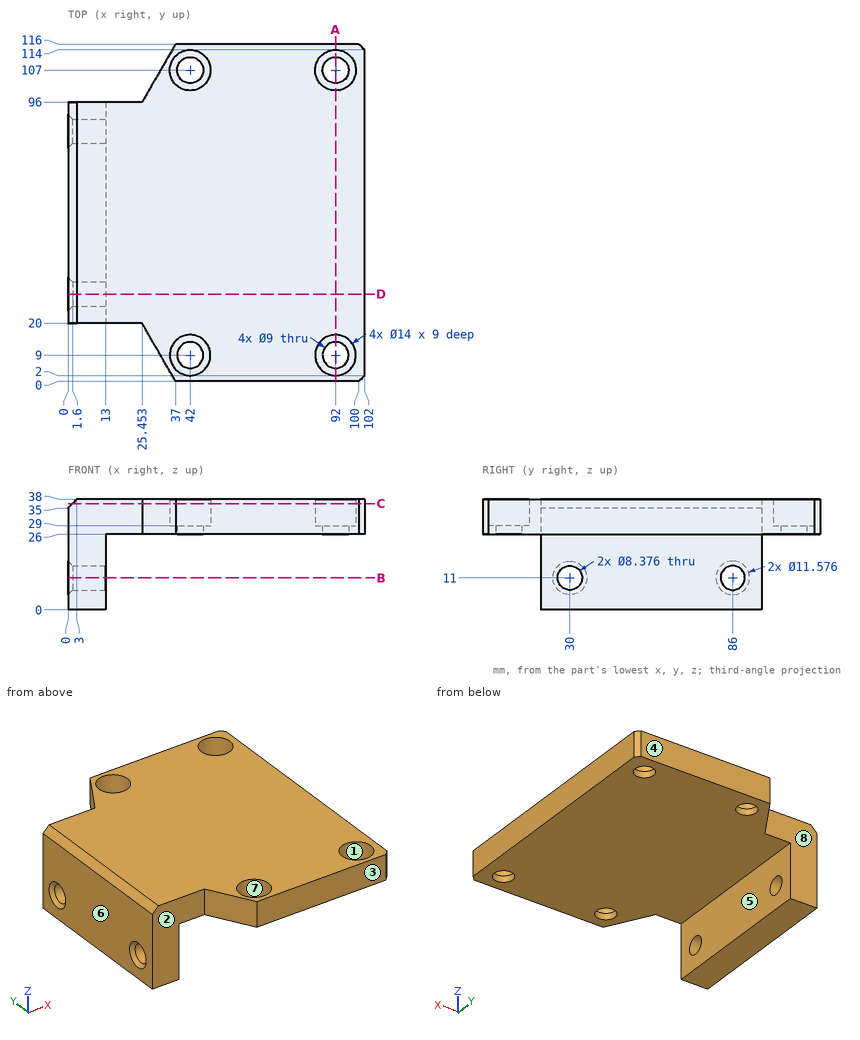
Part print with two shaded views. Sizes in mm from the minimum x, y, z corner. A direction names the side the tool comes from. Round coordinates to 2 decimals unless told otherwise and drop trailing zeros. Order: outer loops, then holes, each group sorted by start corner. A loop starts at its lowest first (then second) coordinate and runs counter-clockwise, first axis right, second up. Notation, with made-up numbers: (62, 89.5) - (91, 89.5) arc R15 ccw to (91, 110.5) - close; hole circle Ø1 at (-12.5, 24.25). An arc over 180 degrees is marked (long way). Answer as CSV lines item,"result". Start each with the question number.
1. Pin check, flat tips, straight feed: pin 1 (12.5 mm diameter, centred on x = 92, y = 107, fed in from +Z); pin 2 (10 mm diameter, centred on y = 56.5, z = 24.5, fed in from +X); pin 3 (13 mm diameter, centred on y = 61.5, z = 9, fed in from +X); pin 4 (14.5 mm diameter, centred on x = 42, y = 9, fed in from -Z). Stop position of each tip, or through.
2. Saw through at B-B, the plane z = 11. Write the cut outline in (x, y), and give its area (3 significant figures).
3. Tool access for the marked faces 1, 2, 3, 4 and 5: list every direction of +Z, -Z, +X, -X, +Y, -Y with a clear straight run to the whole face (end or side of a thin tool).
4. Saw through at A-A, the plane x = 92. Write the cut outline in (y, z).
5. Saw through at C-C, the plane z = 36.5. Write the cut outline in (x, y).
6. Saw through at D-D, the plane y = 30. Write the cut outline in (x, z).
7. Pull direction Y, two halves, no side cores. Call the marked faces 6, 7 and 8: +Y half, -Y half, draft (parallel to the pull), parting line (faces both ways), or undercut.
8. Drill centre lines: L1, parallel to Y at x = 42, z = 26.85; L2, parallel to Y at x = 8, z = 11; L3, parallel to X at y = 107, z = 35.25. Where is each one in solid material? Low to high. Write a range as [from, to].
Model answer:
1,pin 1,"stops at z = 29"
1,pin 2,"stops at x = 102"
1,pin 3,"stops at x = 13"
1,pin 4,"stops at z = 26"
2,outline,"(0, 20) - (13, 20) - (13, 25.81) - (1.6, 25.81) - (0, 24.21) - close; (0, 35.79) - (1.6, 34.19) - (13, 34.19) - (13, 81.81) - (1.6, 81.81) - (0, 80.21) - close; (0, 91.79) - (1.6, 90.19) - (13, 90.19) - (13, 96) - (0, 96) - close"
2,area,"765 mm²"
3,face 1,"+Z"
3,face 2,"+Z, -Z, -X, -Y"
3,face 3,"+Z, -Z, +X, -X, -Y"
3,face 4,"+Z, -Z, +X, -X, +Y"
3,face 5,"-Z, +X, +Y, -Y"
4,outline,"(0, 26) - (4.5, 26) - (4.5, 29) - (2, 29) - (2, 38) - (0, 38) - close; (13.5, 26) - (102.5, 26) - (102.5, 29) - (100, 29) - (100, 38) - (16, 38) - (16, 29) - (13.5, 29) - close; (111.5, 26) - (116, 26) - (116, 38) - (114, 38) - (114, 29) - (111.5, 29) - close"
5,outline,"(1.5, 20) - (25.45, 20) - (37, 0) - (100, 0) - (102, 2) - (102, 114) - (100, 116) - (37, 116) - (25.45, 96) - (1.5, 96) - close; hole circle Ø14 at (42, 9); hole circle Ø14 at (42, 107); hole circle Ø14 at (92, 9); hole circle Ø14 at (92, 107)"
6,outline,"(0, 0) - (13, 0) - (13, 6.81) - (1.6, 6.81) - (0, 5.21) - close; (0, 16.79) - (1.6, 15.19) - (13, 15.19) - (13, 26) - (102, 26) - (102, 38) - (3, 38) - (0, 35) - close"
7,face 6,"draft"
7,face 7,"undercut"
7,face 8,"+Y half"
8,L1,"y = [0, 4.5], [13.5, 102.5], [111.5, 116]"
8,L2,"y = [20, 25.81], [34.19, 81.81], [90.19, 96]"
8,L3,"x = [31.8, 35], [49, 85], [99, 102]"
